Geometry check sheet. Reference: the model listing, model coordinates, mm. Coordinates: 2 decimals unless noted, no trailing zeros. Write each loop counter-clockwise with the first axis right and the second up, starting at its lowest first coordinate (ties: lowest second). Pieces come first, ordered by that corner, then holes.
from build123d import *

# Parameters (mm, degrees)
F1_DEPTH  = 25.4
F2_DEPTH  = 3.175
F3_COUNT  = 17
F1_FACE_R = 9.017
F3_FACE_R = 9.017
F4_DEPTH  = 25.4


with BuildPart() as f1:
    # F0 (on Top) → F1 (new body)
    with BuildSketch(Plane.XY):
        with BuildLine():
            ThreePointArc((9.017, 60.96), (6.375981846, 67.335981846), (0, 69.977))
            Line((0, 69.977), (0, 51.943))
            ThreePointArc((0, 51.943), (6.375981846, 54.584018154), (9.017, 60.96))
        make_face()
        with BuildLine():
            Line((0, 51.943), (0, 69.977))
            ThreePointArc((0, 69.977), (-9.017, 60.96), (0, 51.943))
        make_face()
    extrude(amount=F1_DEPTH)


with BuildPart() as f2:
    # F0 (on Top) → F2 (new body)
    with BuildSketch(Plane.XY):
        with BuildLine():
            ThreePointArc((0, 76.2), (-53.8815367264, -53.8815367264), (76.2, 0))
            ThreePointArc((76.2, 0), (53.8815367264, 53.8815367264), (0, 76.2))
        make_face()
        with BuildLine():
            ThreePointArc((1.5875, 0), (-1.1225320151, -1.1225320151), (0, 1.5875))
            ThreePointArc((0, 1.5875), (1.1225320151, 1.1225320151), (1.5875, 0))
        make_face(mode=Mode.SUBTRACT)
        with BuildLine():
            ThreePointArc((0, 51.943), (-9.017, 60.96), (0, 69.977))
            ThreePointArc((0, 69.977), (6.375981846, 67.335981846), (9.017, 60.96))
            ThreePointArc((9.017, 60.96), (6.375981846, 54.584018154), (0, 51.943))
        make_face(mode=Mode.SUBTRACT)
    extrude(amount=F2_DEPTH)


with BuildPart() as f3_1:
    # F3: instance of F1
    add(f1.part.rotate(Axis((0, 0, 3.175), (0, 0, -1)), 1 * 360 / F3_COUNT))


with BuildPart() as f3_2:
    # F3: instance of F1
    add(f1.part.rotate(Axis((0, 0, 3.175), (0, 0, -1)), 2 * 360 / F3_COUNT))


with BuildPart() as f3_3:
    # F3: instance of F1
    add(f1.part.rotate(Axis((0, 0, 3.175), (0, 0, -1)), 3 * 360 / F3_COUNT))


with BuildPart() as f3_4:
    # F3: instance of F1
    add(f1.part.rotate(Axis((0, 0, 3.175), (0, 0, -1)), 4 * 360 / F3_COUNT))


with BuildPart() as f3_5:
    # F3: instance of F1
    add(f1.part.rotate(Axis((0, 0, 3.175), (0, 0, -1)), 5 * 360 / F3_COUNT))


with BuildPart() as f3_6:
    # F3: instance of F1
    add(f1.part.rotate(Axis((0, 0, 3.175), (0, 0, -1)), 6 * 360 / F3_COUNT))


with BuildPart() as f3_7:
    # F3: instance of F1
    add(f1.part.rotate(Axis((0, 0, 3.175), (0, 0, -1)), 7 * 360 / F3_COUNT))


with BuildPart() as f3_8:
    # F3: instance of F1
    add(f1.part.rotate(Axis((0, 0, 3.175), (0, 0, -1)), 8 * 360 / F3_COUNT))


with BuildPart() as f3_9:
    # F3: instance of F1
    add(f1.part.rotate(Axis((0, 0, 3.175), (0, 0, -1)), 9 * 360 / F3_COUNT))


with BuildPart() as f3_10:
    # F3: instance of F1
    add(f1.part.rotate(Axis((0, 0, 3.175), (0, 0, -1)), 10 * 360 / F3_COUNT))


with BuildPart() as f3_11:
    # F3: instance of F1
    add(f1.part.rotate(Axis((0, 0, 3.175), (0, 0, -1)), 11 * 360 / F3_COUNT))


with BuildPart() as f3_12:
    # F3: instance of F1
    add(f1.part.rotate(Axis((0, 0, 3.175), (0, 0, -1)), 12 * 360 / F3_COUNT))


with BuildPart() as f3_13:
    # F3: instance of F1
    add(f1.part.rotate(Axis((0, 0, 3.175), (0, 0, -1)), 13 * 360 / F3_COUNT))


with BuildPart() as f3_14:
    # F3: instance of F1
    add(f1.part.rotate(Axis((0, 0, 3.175), (0, 0, -1)), 14 * 360 / F3_COUNT))


with BuildPart() as f3_15:
    # F3: instance of F1
    add(f1.part.rotate(Axis((0, 0, 3.175), (0, 0, -1)), 15 * 360 / F3_COUNT))


with BuildPart() as f3_16:
    # F3: instance of F1
    add(f1.part.rotate(Axis((0, 0, 3.175), (0, 0, -1)), 16 * 360 / F3_COUNT))


with BuildPart() as f4_tool:
    # F1_face (on face) + F3_face (on face) → F4 (new body)
    with BuildSketch(Plane(origin=(0, 60.96, 25.4), x_dir=(1, 0, 0), z_dir=(0, 0, 1))):
        Circle(F1_FACE_R)
    with BuildSketch(Plane(origin=(22.0212919708, 56.8435071045, 25.4), x_dir=(1, 0, 0), z_dir=(0, 0, 1))):
        Circle(F3_FACE_R)
        with Locations((19.0471944659, -11.7935235107)):
            Circle(F3_FACE_R)
        with Locations((32.5478622702, -29.6712969364)):
            Circle(F3_FACE_R)
        with Locations((38.6786634162, -51.2188279116)):
            Circle(F3_FACE_R)
        with Locations((36.611599237, -73.5260029793)):
            Circle(F3_FACE_R)
        with Locations((26.6258382042, -93.5801145382)):
            Circle(F3_FACE_R)
        with Locations((10.0700126782, -108.6727436986)):
            Circle(F3_FACE_R)
        with Locations((-10.8199213647, -116.7655472612)):
            Circle(F3_FACE_R)
        with Locations((-33.2226625769, -116.7655472612)):
            Circle(F3_FACE_R)
        with Locations((-22.0212919708, 4.1164928955)):
            Circle(F3_FACE_R)
        with Locations((-44.0425839415, 0)):
            Circle(F3_FACE_R)
        with Locations((-63.0897784075, -11.7935235107)):
            Circle(F3_FACE_R)
        with Locations((-76.5904462118, -29.6712969364)):
            Circle(F3_FACE_R)
        with Locations((-80.6541831786, -73.5260029793)):
            Circle(F3_FACE_R)
        with Locations((-70.6684221458, -93.5801145382)):
            Circle(F3_FACE_R)
        with Locations((-54.1125966198, -108.6727436986)):
            Circle(F3_FACE_R)
        with Locations((-82.7212473577, -51.2188279116)):
            Circle(F3_FACE_R)
    extrude(amount=-F4_DEPTH)


with BuildPart() as f1_1:
    add(f1.part)

    # F4: cut by f4_tool
    add(f4_tool.part, mode=Mode.SUBTRACT)


with BuildPart() as f2_1:
    add(f2.part)

    # F4: cut by f4_tool
    add(f4_tool.part, mode=Mode.SUBTRACT)


with BuildPart() as f3_1_1:
    add(f3_1.part)

    # F4: cut by f4_tool
    add(f4_tool.part, mode=Mode.SUBTRACT)


with BuildPart() as f3_2_1:
    add(f3_2.part)

    # F4: cut by f4_tool
    add(f4_tool.part, mode=Mode.SUBTRACT)


with BuildPart() as f3_3_1:
    add(f3_3.part)

    # F4: cut by f4_tool
    add(f4_tool.part, mode=Mode.SUBTRACT)


with BuildPart() as f3_4_1:
    add(f3_4.part)

    # F4: cut by f4_tool
    add(f4_tool.part, mode=Mode.SUBTRACT)


with BuildPart() as f3_5_1:
    add(f3_5.part)

    # F4: cut by f4_tool
    add(f4_tool.part, mode=Mode.SUBTRACT)


with BuildPart() as f3_6_1:
    add(f3_6.part)

    # F4: cut by f4_tool
    add(f4_tool.part, mode=Mode.SUBTRACT)


with BuildPart() as f3_7_1:
    add(f3_7.part)

    # F4: cut by f4_tool
    add(f4_tool.part, mode=Mode.SUBTRACT)


with BuildPart() as f3_8_1:
    add(f3_8.part)

    # F4: cut by f4_tool
    add(f4_tool.part, mode=Mode.SUBTRACT)


with BuildPart() as f3_9_1:
    add(f3_9.part)

    # F4: cut by f4_tool
    add(f4_tool.part, mode=Mode.SUBTRACT)


with BuildPart() as f3_10_1:
    add(f3_10.part)

    # F4: cut by f4_tool
    add(f4_tool.part, mode=Mode.SUBTRACT)


with BuildPart() as f3_11_1:
    add(f3_11.part)

    # F4: cut by f4_tool
    add(f4_tool.part, mode=Mode.SUBTRACT)


with BuildPart() as f3_12_1:
    add(f3_12.part)

    # F4: cut by f4_tool
    add(f4_tool.part, mode=Mode.SUBTRACT)


with BuildPart() as f3_13_1:
    add(f3_13.part)

    # F4: cut by f4_tool
    add(f4_tool.part, mode=Mode.SUBTRACT)


with BuildPart() as f3_14_1:
    add(f3_14.part)

    # F4: cut by f4_tool
    add(f4_tool.part, mode=Mode.SUBTRACT)


with BuildPart() as f3_15_1:
    add(f3_15.part)

    # F4: cut by f4_tool
    add(f4_tool.part, mode=Mode.SUBTRACT)


with BuildPart() as f3_16_1:
    add(f3_16.part)

    # F4: cut by f4_tool
    add(f4_tool.part, mode=Mode.SUBTRACT)


solid = f2_1.part
1. Sectioned sample at B-B, the plane x = 29. Record the boundary of the cut face in (y, z) (1 decimal).
Computed values:
outline: (-70.5, 0) - (-60.3, 0) - (-60.3, 3.2) - (-70.5, 3.2) - close; (-43.4, 0) - (51.1, 0) - (51.1, 3.2) - (-43.4, 3.2) - close; (62.6, 0) - (70.5, 0) - (70.5, 3.2) - (62.6, 3.2) - close
2. Gauge pin test, flat ends, axial feed: pin 1 Ø11 at (x, y) = (32.09, -51.83) entering from -Z; pin 2 Ø1.5 at (x, z) = (45, 2) entering from +Y. Record the tip position at first contact, or that the pin passes through.
Computed values:
pin 1: passes through
pin 2: stops at y = 62.04
3. Sectioned sample at A-A, the plane y = -64. Record the boundary of the cut face in (x, z) (3 decimals).
Computed values:
outline: (-41.357, 0) - (-19.244, 0) - (-19.244, 3.175) - (-41.357, 3.175) - close; (-3.159, 0) - (3.159, 0) - (3.159, 3.175) - (-3.159, 3.175) - close; (19.244, 0) - (41.357, 0) - (41.357, 3.175) - (19.244, 3.175) - close
4. Draft check along Y on faces 1 (the cylindrical face through (-67.64, -16.29, 1.61)), 2 (the flat face through (-1, -16, 3.175)), 3 (the cylindrical face through (-60.47, -46.367, 1.565)). Enter one of: released by +Y, released by -Y, zero draft, split by the parting line, or undercut.
Computed values:
face 1: undercut
face 2: zero draft
face 3: split by the parting line
5. Sectioned sample at C-C, the plane z = 1.3. Give the number of separate pieces and of enclosed holes in the cut face, and give its area (3 significant figures).
Computed values:
separate pieces: 1
enclosed holes: 18
area: 13,900 mm2
6. Thickness scan on line 1 along X through (y, z) = (43.5, 2); line 2 along Y through (x, z) = (36.5, 1.55); line 3 along X through (y, z) = (25, 2.9). Record the ranges inside material, lowest first.
Computed values:
line 1: x = -62.56 to -49.95, -32.19 to 32.19, 49.95 to 62.56
line 2: y = -66.89 to -59.69, -43.96 to 37.28, 52.82 to 66.89
line 3: x = -71.98 to -63.32, -45.82 to 45.82, 63.32 to 71.98
